Geometry check sheet. Reference: the model listing, model coordinates, mm. A direction names the side the tool comes from. Coordinates: 2 decimals unless noted, no trailing zeros. Loops run counter-clockwise (first coordinate to the right, second up) from the corner with the lowest first, then second, coordinate; pieces in that order, holes last. Notation, with made-up numbers: (-2, -39.75) - (3, -39.75) arc R25 ccw to (3, -4.75) - close; hole circle Ø1 at (25, -16.5). An arc over 180 degrees is marked (long way). One line per item, written item: value.
from build123d import *

# Parameters (mm, degrees)
BOSS_EXTRUDE1_DEPTH                              = 10
SKETCH2_W                                        = 16
SKETCH2_H                                        = 18
CBORE_FOR_M4_HEX_HEAD_MACHINE_SCREW1_D           = 4.5
CBORE_FOR_M4_HEX_HEAD_MACHINE_SCREW1_DEPTH       = 26
CBORE_FOR_M4_HEX_HEAD_MACHINE_SCREW1_CBORE_D     = 8
CBORE_FOR_M4_HEX_HEAD_MACHINE_SCREW1_CBORE_DEPTH = 4.5
CHAMFER1_SIZE                                    = 0.36
FILLET1_R                                        = 0.3


with BuildPart() as part:
    # Sketch1 → Boss-Extrude1 (new body)
    with BuildSketch(Plane(origin=(16, 0, 0), x_dir=(0, -1, 0), z_dir=(-1, 0, 0))):
        with BuildLine():
            Line((15.652475842, 22), (-15.652475842, 22))
            ThreePointArc((-15.652475842, 22), (-19.091883092, 19.091883092), (-22, 15.652475842))
            Line((-22, 15.652475842), (-22, -15.652475842))
            ThreePointArc((-22, -15.652475842), (-19.091883092, -19.091883092), (-15.652475842, -22))
            Line((-15.652475842, -22), (15.652475842, -22))
            ThreePointArc((15.652475842, -22), (19.091883092, -19.091883092), (22, -15.652475842))
            Line((22, -15.652475842), (22, 15.652475842))
            ThreePointArc((22, 15.652475842), (19.091883092, 19.091883092), (15.652475842, 22))
        make_face()
    extrude(amount=-BOSS_EXTRUDE1_DEPTH)

    # Sketch2 → Revolve1 (revolve)
    with BuildSketch(Plane.XY, mode=Mode.PRIVATE) as revolve1_sk:
        with Locations((8, 9)):
            Rectangle(SKETCH2_W, SKETCH2_H)
    revolve(revolve1_sk.sketch.rotate(Axis((0, 0, 0), (1, 0, 0)), 270), axis=Axis((0, 0, 0), (1, 0, 0)))

    # Sketch3 → Cut-Revolve1 (revolve, cut)
    with BuildSketch(Plane.XY, mode=Mode.PRIVATE) as cut_revolve1_sk:
        Polygon((0, 7.75), (0, 0), (26, 0), (26, 15), (21, 15), (21, 14), (5, 14), (5, 7.75), align=None)
    revolve(cut_revolve1_sk.sketch.rotate(Axis((0, 0, 0), (1, 0, 0)), 270), axis=Axis((0, 0, 0), (1, 0, 0)), mode=Mode.SUBTRACT)

    # CBORE for M4 Hex Head Machine Screw1
    with Locations(Plane(origin=(26, 0, 0), x_dir=(0, 0, -1), z_dir=(1, 0, 0))):
        with Locations((-15.556349186, -15.556349186), (15.556349186, 15.556349186), (15.556349186, -15.556349186), (-15.556349186, 15.556349186)):
            CounterBoreHole(CBORE_FOR_M4_HEX_HEAD_MACHINE_SCREW1_D / 2, CBORE_FOR_M4_HEX_HEAD_MACHINE_SCREW1_CBORE_D / 2, CBORE_FOR_M4_HEX_HEAD_MACHINE_SCREW1_CBORE_DEPTH, depth=CBORE_FOR_M4_HEX_HEAD_MACHINE_SCREW1_DEPTH)

    # Chamfer1
    chamfer1_edges = [part.edges().sort_by_distance(p)[0] for p in [
        (26, 19.091883092, 19.091883092),
        (16, -19.091883092, 19.091883092),
        (26, 19.091883092, -19.091883092),
        (26, -19.091883092, -19.091883092),
        (0, 0, 18),
        (26, -19.091883092, 19.091883092),
        (16, -19.091883092, -19.091883092),
        (16, 19.091883092, -19.091883092),
        (16, 19.091883092, 19.091883092),
    ]]
    chamfer(chamfer1_edges, length=CHAMFER1_SIZE)

    # Fillet1
    fillet1_edges = [part.edges().sort_by_distance(p)[0] for p in [
        (16, 0, 18),
    ]]
    fillet(fillet1_edges, radius=FILLET1_R)


solid = part.part
(1) Material ranges on probe 1 along Z at (x, y) = (23.25, 16); probe 2 along Y at (x, z) = (23.75, 12.5); probe 3 along Y at (x, z) = (18.25, 16.5), recorded low to high. Write a range as from..to.
Reply:
probe 1: -21.75..-19.53, -11.58..11.58, 19.53..21.75
probe 2: -22..-18.14, -12.98..-8.29, 8.29..12.98, 18.14..22
probe 3: -21.37..-17.6, -13.51..13.51, 17.6..21.37
(2) Cross-section at D-D on x = 18.5. Record the cut outline in (y, z).
Reply:
outline: (-22, -15.65) arc R27 ccw to (-15.65, -22) - (15.65, -22) arc R27 ccw to (22, -15.65) - (22, 15.65) arc R27 ccw to (15.65, 22) - (-15.65, 22) arc R27 ccw to (-22, 15.65) - close; hole circle Ø4.5 at (-15.56, -15.56); hole circle Ø4.5 at (-15.56, 15.56); hole circle Ø28 at (0, 0); hole circle Ø4.5 at (15.56, -15.56); hole circle Ø4.5 at (15.56, 15.56)
(3) Release check for a two-part mould opening along Z. For faces 4 (the face through (20.935, -19.136, 19.047)), 5 (the face through (23.78, -15.38, -11.56)), 6 (the face through (0, -4, 8)) record: pulls with the +Z half, pulls with the -Z half, needs draft (parallel to the pull), parting line crosses it, or undercut.
Reply:
face 4: pulls with the +Z half
face 5: undercut
face 6: needs draft
(4) Cross-section at C-C on x = 6. Record the cut outline in (y, z).
Reply:
outline: circle Ø36 at (0, 0); hole circle Ø28 at (0, 0)
(5) Access from +Z, -Z, +X, -X, +Y, -Y to the whole of each face (thin tool, end or side, straight path). Record for faces 1 (the face through (16.143, 18.987, -18.889)), 2 (the face through (23.782, 15.732, 19.552)), 3 (the face through (16, -5, -18)).
Reply:
face 1: -Z, -X, +Y
face 2: +X
face 3: -X
(6) Cross-section at A-A on y = 0. Record the cut outline in (x, z), and give its area (3 significant figures).
Reply:
outline: (0, -17.64) - (0.36, -18) - (15.7, -18) arc R0.3 cw to (16, -18.3) - (16, -22) - (26, -22) - (26, -15) - (21, -15) - (21, -14) - (5, -14) - (5, -7.75) - (0, -7.75) - close; (0, 7.75) - (5, 7.75) - (5, 14) - (21, 14) - (21, 15) - (26, 15) - (26, 22) - (16, 22) - (16, 18.3) arc R0.3 cw to (15.7, 18) - (0.36, 18) - (0, 17.64) - close
area: 340 mm2
(7) Go/stop test with flat-tipped pins: pin 1 Ø7 at (y, z) = (15.56, -15.56) entering from -X; pin 2 Ø4 at (y, z) = (16, -15) entering from +X; pin 3 Ø4 at (x, z) = (6, 2) entering from -Y. Record where each tip stops, or that it passes through.
Reply:
pin 1: x = 16
pin 2: x = 21.5
pin 3: y = -18
